The model under review builds one solid part; all positions refer to its coordinate system, in mm. A direction names the side the tool comes from. Give positions to 0.01 mm unless a question says otherwise; leave off trailing zeros. Order: outer loops, then holes, each group sorted by start corner. A loop starts at its lowest first (then second) coordinate and runs counter-clockwise, first axis right, second up. Notation, with made-up numbers: (38.5, 41) -> (83.5, 41) arc R12 ccw to (83.5, 46) -> close; hole circle Ø10 at (69, -27). An arc over 180 degrees is marked (long way). Answer as a JSON object with one key per item and string values. Group by question number.
from build123d import *

# Parameters (mm, degrees)
F0_W            = 100.3
F0_H            = 100.3
F1_DEPTH        = 9.13
F2_SIZE         = 2
F4_D            = 4.5
F4_CBORE_D      = 8.2
F4_CBORE_DEPTH  = 4.4
F5_D            = 13
F10_D           = 2.5
F10_DEPTH       = 5.5
F10_TIP         = 0.7510757738
F10_ON_F7_D     = 2.5
F10_ON_F7_DEPTH = 5.5
F10_ON_F7_TIP   = 0.7510757738
F10_ON_F6_D     = 2.5
F10_ON_F6_DEPTH = 5.5
F10_ON_F6_TIP   = 0.7510757738
F10_ON_F9_D     = 2.5
F10_ON_F9_DEPTH = 5.5
F10_ON_F9_TIP   = 0.7510757738


with BuildPart() as f1:
    # F0 (on Front) → F1 (new body)
    with BuildSketch(Plane.XZ):
        Rectangle(F0_W, F0_H)
    extrude(amount=F1_DEPTH)

    # F2
    f2_edges = [f1.edges().sort_by_distance(p)[0] for p in [
        (-50.15, -4.565, -50.15),
        (50.15, -4.565, -50.15),
        (50.15, -4.565, 50.15),
        (-50.15, -4.565, 50.15),
    ]]
    chamfer(f2_edges, length=F2_SIZE)

    # F4 (through all)
    with Locations(Plane.XZ.offset(9.13)):
        with Locations((-36.75, -3.15), (-3.15, -36.75)):
            CounterBoreHole(F4_D / 2, F4_CBORE_D / 2, F4_CBORE_DEPTH)

    # F5 (through all)
    with Locations(Plane.XZ.offset(9.13)):
        with Locations((0, 0)):
            Hole(F5_D / 2)

    # F10
    with Locations(Plane(origin=(-50.15, 0, 0), x_dir=(0, -1, 0), z_dir=(-1, 0, 0))):
        with Locations((4.5, -30), (4.5, 30)):
            Hole(F10_D / 2, depth=F10_DEPTH)
            with Locations((0, 0, -(F10_DEPTH + F10_TIP / 2))):  # 118° drill point
                Cone(0, F10_D / 2, F10_TIP, mode=Mode.SUBTRACT)

    # F10 on F7
    with Locations(Plane.XY.offset(50.15)):
        with Locations((-30, -4.5), (30, -4.5)):
            Hole(F10_ON_F7_D / 2, depth=F10_ON_F7_DEPTH)
            with Locations((0, 0, -(F10_ON_F7_DEPTH + F10_ON_F7_TIP / 2))):  # 118° drill point
                Cone(0, F10_ON_F7_D / 2, F10_ON_F7_TIP, mode=Mode.SUBTRACT)

    # F10 on F6
    with Locations(Plane.YZ.offset(50.15)):
        with Locations((-4.5, -30), (-4.5, 30)):
            Hole(F10_ON_F6_D / 2, depth=F10_ON_F6_DEPTH)
            with Locations((0, 0, -(F10_ON_F6_DEPTH + F10_ON_F6_TIP / 2))):  # 118° drill point
                Cone(0, F10_ON_F6_D / 2, F10_ON_F6_TIP, mode=Mode.SUBTRACT)

    # F10 on F9
    with Locations(Plane(origin=(0, 0, -50.15), x_dir=(1, 0, 0), z_dir=(0, 0, -1))):
        with Locations((30, 4.5), (-30, 4.5)):
            Hole(F10_ON_F9_D / 2, depth=F10_ON_F9_DEPTH)
            with Locations((0, 0, -(F10_ON_F9_DEPTH + F10_ON_F9_TIP / 2))):  # 118° drill point
                Cone(0, F10_ON_F9_D / 2, F10_ON_F9_TIP, mode=Mode.SUBTRACT)


solid = f1.part
1. Take a section at B-B on z = -3.15. Give the boundary of the cut face in (x, y), plus the area to 3 significant figures.
2. Take a section at A-A on y = -1.5. Give the boundary of the cut face in (x, z).
3. Draft analysis for pull direction Y (two halves, no side actions). For faces 1 (the flat face through (-1, -5, -50.15)), 2 (the cylindrical face through (28.845, -4.021, -47.362)), 3 (the flat face through (-1, -4.73, -39)), state which applies: pulls with the +Y half, pulls with the -Y half, needs draft (parallel to the pull), parting line crosses it, or undercut.
4. Take a section at C-C on x = -3.15. Give the boundary of the cut face in (y, z), plus the area to 3 significant figures.
5. Machinability: for faces 4 (the cylindrical face through (-40.846, -6.961, -2.97)), 5 (the cylindrical face through (47.362, -5.172, -28.946)), 6 (the flat face through (-1, -5, 50.15)), 7 (the cylindrical face through (-47.362, -3.828, -28.946)), 8 (the cylindrical face through (-31.155, -4.979, 47.362)), which of the approach directions +Z, -Z, +X, -X, +Y, -Y give a long, thin tool a straight path to every point of the face, cutting with its end or side? Answer none if there is none.
6. For probe 1 along Z at (x, y) = (47.2, -4.5); probe 2 along Z at (x, y) = (-5, -0.75); probe 3 along X at (y, z) = (-4.5, -49), list the stretches that pass through material, from the lowest coordinate up. Write a range as [from, to].
7. For pin 1 (10 mm diameter, centred on x = 11.5, z = -22, fed in from +Y); pin 2 (5 mm diameter, centred on x = -3.15, z = -36.75, fed in from -Y); pin 3 (10.5 mm diameter, centred on x = 0, z = 0, fed in from -Y); pin 4 (1.5 mm diameter, centred on x = 30, y = -4.5, fed in from +Z), all flat-tipped, find the tip position at first contact; note any pin that passes through.
Checks:
{
 "1": {"outline": "(-50.15, -9.13) -> (-40.85, -9.13) -> (-40.85, -4.73) -> (-39, -4.73) -> (-39, 0) -> (-50.15, 0) -> close; (-34.5, -4.73) -> (-32.65, -4.73) -> (-32.65, -9.13) -> (-5.69, -9.13) -> (-5.69, 0) -> (-34.5, 0) -> close; (5.69, -9.13) -> (50.15, -9.13) -> (50.15, 0) -> (5.69, 0) -> close", "area": "755 mm2"},
 "2": {"outline": "(-50.15, -48.15) -> (-48.15, -50.15) -> (48.15, -50.15) -> (50.15, -48.15) -> (50.15, 48.15) -> (48.15, 50.15) -> (-48.15, 50.15) -> (-50.15, 48.15) -> close; hole circle Ø4.5 at (-36.75, -3.15); hole circle Ø13 at (0, 0); hole circle Ø4.5 at (-3.15, -36.75)"},
 "3": {"face 1": "needs draft", "face 2": "undercut", "face 3": "pulls with the -Y half"},
 "4": {"outline": "(-9.13, -50.15) -> (0, -50.15) -> (0, -39) -> (-4.73, -39) -> (-4.73, -40.85) -> (-9.13, -40.85) -> close; (-9.13, -32.65) -> (-4.73, -32.65) -> (-4.73, -34.5) -> (0, -34.5) -> (0, -5.69) -> (-9.13, -5.69) -> close; (-9.13, 5.69) -> (0, 5.69) -> (0, 50.15) -> (-9.13, 50.15) -> close", "area": "755 mm2"},
 "5": {"face 4": "-Y", "face 5": "+X", "face 6": "+Z, +X, -X, +Y, -Y", "face 7": "-X", "face 8": "+Z"},
 "6": {"probe 1": "z = [-50.15, -31.25], [-28.75, 28.75], [31.25, 50.15]", "probe 2": "z = [-50.15, -38.03], [-35.47, -4.15], [4.15, 50.15]", "probe 3": "x = [-49.3, -31.25], [-28.75, 28.75], [31.25, 49.3]"},
 "7": {"pin 1": "stops at y = 0", "pin 2": "stops at y = -4.73", "pin 3": "passes through", "pin 4": "stops at z = 44.35"}
}
